Can you work these out from the model? Positions are in its coordinate system, mm. Face numbers are marked on the shaded views. A direction names the side the tool comes from. Give positions to 0.01 mm unless a question says otherwise; leave off trailing zeros. Order: outer loops, then holes, each group sorted by start corner. A loop starts at its lowest first (then second) coordinate and runs counter-clockwise, first axis right, second up. Notation, with made-up numbers: (12.25, 34) -> (52.25, 34) arc R27 cw to (52.25, 72) -> close; hole circle Ø11 at (-29.75, 81). An arc over 180 degrees is marked (long way). Answer as a JSON object with one key per item and string values.
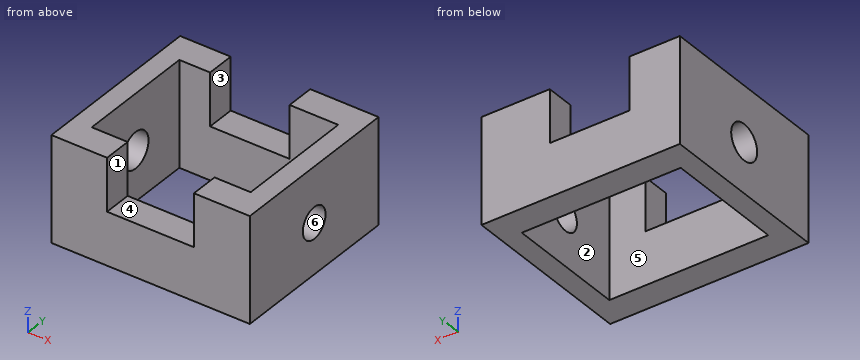
```python
from build123d import *

# Parameters (mm, degrees)
F0_W      = 95.6981405616
F0_H      = 85.2225497365
F0_W_2    = 76.6617953777
F0_H_2    = 57.9620860517
F1_DEPTH  = 50.8
F2_W      = 41.8984405696
F2_H      = 13.6302318424
F4_DEPTH  = 25.4
F5_W      = 38.359541446
F5_H      = 13.6302318424
F6_DEPTH  = 25.4
F7_R      = 7.5298291719
F8_DEPTH  = 38.1
F9_R      = 7.8998800408
F10_DEPTH = 38.1
F11_R     = 8.5919528165
F12_DEPTH = 25.4


with BuildPart() as f1:
    # F0 (on Top) → F1 (new body)
    with BuildSketch(Plane.XY):
        Rectangle(F0_W, F0_H)
        Rectangle(F0_W_2, F0_H_2, mode=Mode.SUBTRACT)
    extrude(amount=F1_DEPTH)

    # F2 (on face) → F4 (cut)
    with BuildSketch(Plane.XY.offset(50.8)):
        with Locations((-0.0701360404, -35.7961589471)):
            Rectangle(F2_W, F2_H)
    extrude(amount=-F4_DEPTH, mode=Mode.SUBTRACT)

    # F5 (on face) → F6 (cut)
    with BuildSketch(Plane.XY.offset(50.8)):
        with Locations((-4.2936895043, 35.7961589471)):
            Rectangle(F5_W, F5_H)
    extrude(amount=-F6_DEPTH, mode=Mode.SUBTRACT)

    # F7 (on face) → F8 (cut)
    with BuildSketch(Plane.YZ.offset(47.8490702808)):
        with Locations((0, 24.2426600307)):
            Circle(F7_R)
    extrude(amount=-F8_DEPTH, mode=Mode.SUBTRACT)

    # F9 (on face) → F10 (cut)
    with BuildSketch(Plane(origin=(-47.8490702808, 0, 0), x_dir=(0, -1, 0), z_dir=(-1, 0, 0))):
        with Locations((0, 24.427017197)):
            Circle(F9_R)
    extrude(amount=F10_DEPTH, mode=Mode.SUBTRACT)

    # F11 (on face) → F12 (cut)
    with BuildSketch(Plane(origin=(-47.8490702808, 0, 0), x_dir=(0, -1, 0), z_dir=(-1, 0, 0))):
        with Locations((0, 24.0862686187)):
            Circle(F11_R)
    extrude(amount=-F12_DEPTH, mode=Mode.SUBTRACT)


solid = f1.part
```
1. Will these pins go through, and if not, where does the flat tip stop? pin 1 Ø6 at (x, y) = (-28.5, 28.5) entering from -Z; pin 2 Ø7 at (x, y) = (-6.5, 34) entering from +Z.
Worked answers:
{"pin 1": "z = 0", "pin 2": "z = 25.4"}
2. If we section it at A-A on y = 0: Please give me the cut outline in (x, z), then the cut area to 3 significant figures.
Worked answers:
{"outline": "(-47.85, 0) -> (-38.33, 0) -> (-38.33, 15.49) -> (-47.85, 15.49) -> close; (-47.85, 32.68) -> (-38.33, 32.68) -> (-38.33, 50.8) -> (-47.85, 50.8) -> close; (38.33, 0) -> (47.85, 0) -> (47.85, 16.71) -> (38.33, 16.71) -> close; (38.33, 31.77) -> (47.85, 31.77) -> (47.85, 50.8) -> (38.33, 50.8) -> close", "area": "660 mm²"}
3. If we section it at B-B on x = -10.5: Please give me the cut outline in (y, z).
Worked answers:
{"outline": "(-42.61, 0) -> (-28.98, 0) -> (-28.98, 25.4) -> (-42.61, 25.4) -> close; (28.98, 0) -> (42.61, 0) -> (42.61, 25.4) -> (28.98, 25.4) -> close"}
4. Please list where these lines run through material, in increasing order: L1, parallel to Z at x = 45.75, y = 0; L2, parallel to X at y = -18, z = 31; L3, parallel to Z at x = -45.5, y = 0.
Worked answers:
{"L1": "0 to 16.71, 31.77 to 50.8", "L2": "-47.85 to -38.33, 38.33 to 47.85", "L3": "0 to 15.49, 32.68 to 50.8"}
5. For the marked faces 1, 2 and 3, which set-ups out of +Z, -Z, +X, -X, +Y, -Y let a thin tool reach every point of the face, with its end or its side?
Worked answers:
{"face 1": "+Z, +Y, -Y", "face 2": "+Z, -Z", "face 3": "+Z, +Y"}
6. If we section it at D-D on z = 5.5: Please give me the cut outline in (x, y).
Worked answers:
{"outline": "(-47.85, -42.61) -> (47.85, -42.61) -> (47.85, 42.61) -> (-47.85, 42.61) -> close; hole (-38.33, -28.98) -> (38.33, -28.98) -> (38.33, 28.98) -> (-38.33, 28.98) -> close"}
7. If we mould it in two halves opening along Z, with no side actions, what happens to the marked faces 4, 5 and 6? For each: +Z half, -Z half, draft (parallel to the pull), parting line (faces both ways), or undercut.
Worked answers:
{"face 4": "+Z half", "face 5": "draft", "face 6": "undercut"}
8. If we section it at C-C on y = -16.5: Please give me the cut outline in (x, z).
Worked answers:
{"outline": "(-47.85, 0) -> (-38.33, 0) -> (-38.33, 50.8) -> (-47.85, 50.8) -> close; (38.33, 0) -> (47.85, 0) -> (47.85, 50.8) -> (38.33, 50.8) -> close"}
